Read the model definition and answer for the solid it produces. Units are mm, in the model's axes. Face numbers are marked on the shaded views. A direction names the side the tool comes from. Coordinates: 2 decimals unless noted, no trailing zeros. Loops run counter-clockwise (first coordinate to the right, second up) from the corner with the lowest first, then second, coordinate; pieces in that order, holes last. Notation, with made-up numbers: (-36.75, 72) - (-11.75, 72) arc R15 cw to (-11.75, 94) - close; hole circle Ø2 at (59.5, -12). An arc over 180 degrees is marked (long way). Use CSV: the item, a comma, the result in double quotes.
```python
from build123d import *

# Parameters (mm, degrees)
SKETCH3_W               = 6
SKETCH3_H               = 4
BOSS_EXTRUDE4_DEPTH     = 1
SKETCH7_W               = 2.025
SKETCH7_H               = 1
LPATTERN1_COUNT         = 5
LPATTERN1_PITCH         = 3
CUT_EXTRUDE2_DEPTH      = 15.053469323
CUT_EXTRUDE2_DEPTH_BACK = 15.053469323
CUT_EXTRUDE3_REACH      = 29.263
SKETCH6_R               = 1.5
SKETCH8_OUTSIDE_W       = 13.608
SKETCH8_OUTSIDE_H       = 12.19
SKETCH8_OUTSIDE_R       = 3
CUT_EXTRUDE4_DEPTH      = 15.017845865
CUT_EXTRUDE4_DEPTH_BACK = 15.017845865


with BuildPart() as part:
    # Sketch1 → Revolve5 (revolve)
    with BuildSketch(Plane.XY):
        Polygon((0, 13.5), (-2.5, 13.5), (-2.5, 13), (-2, 13), (-2, 5), (-2.25, 5), (-2.25, 4), (-2, 4), (-2, -13), (-2.5, -13), (-2.5, -13.5), (0, -13.5), align=None)
    revolve(axis=Axis((0, 13.5, 0), (0, -1, 0)))

    # Sketch3 → Boss-Extrude4 (add, symmetric)
    with BuildSketch(Plane.XY):
        with Locations((0, 4.5)):
            Rectangle(SKETCH3_W, SKETCH3_H)
    extrude(amount=BOSS_EXTRUDE4_DEPTH, both=True)

    # Sketch7 → Revolve7 (revolve)
    with BuildSketch(Plane.XY, mode=Mode.PRIVATE) as revolve7_sk:
        with Locations((-1.0125, -0.004180602)):
            Rectangle(SKETCH7_W, SKETCH7_H)
    revolve7 = revolve(revolve7_sk.sketch.rotate(Axis((0, 5, 0), (0, -1, 0)), 330), axis=Axis((0, 5, 0), (0, -1, 0)))

    # LPattern1: Revolve7 ×5
    with Locations(*[(0, -i * LPATTERN1_PITCH, 0) for i in range(1, LPATTERN1_COUNT)]):
        add(revolve7)

    # Sketch5 → Cut-Extrude2 (cut, two sides)
    with BuildSketch(Plane.XY) as cut_extrude2_sk:
        with BuildLine():
            Line((-1, 13.5), (-1, 10.5))
            ThreePointArc((-1, 10.5), (0, 9.5), (1, 10.5))
            Line((1, 10.5), (1, 13.5))
            Line((1, 13.5), (-1, 13.5))
        make_face()
        with BuildLine():
            Line((-1, -13.5), (-1, -10.5))
            ThreePointArc((-1, -10.5), (0, -9.5), (1, -10.5))
            Line((1, -10.5), (1, -13.5))
            Line((1, -13.5), (-1, -13.5))
        make_face()
    extrude(amount=CUT_EXTRUDE2_DEPTH, mode=Mode.SUBTRACT)
    extrude(cut_extrude2_sk.sketch, amount=-CUT_EXTRUDE2_DEPTH_BACK, mode=Mode.SUBTRACT)

    # Cut-Extrude3: up to this face of the body (flat: up to its plane)
    cut_extrude3_end = Plane(part.part.faces().sort_by_distance((-1.618726141, -13.5, 0))[0])
    # Sketch6 → Cut-Extrude3 (cut, up to the picked face)
    with BuildSketch(Plane(origin=(0, 13.5, 0), x_dir=(1, 0, 0), z_dir=(0, 1, 0)), mode=Mode.PRIVATE) as cut_extrude3_sk1:
        with Locations(Location((0, 0, 0), (0, 0, 228.189685104))):
            Circle(SKETCH6_R)
    cut_extrude3_tool1 = split(extrude(cut_extrude3_sk1.sketch, amount=-CUT_EXTRUDE3_REACH, mode=Mode.PRIVATE), bisect_by=cut_extrude3_end, keep=Keep.BOTH, mode=Mode.PRIVATE)
    add(cut_extrude3_tool1.solids().sort_by(Axis((0, 13.5, 0), (0, -1, 0)))[0], mode=Mode.SUBTRACT)

    # Sketch8 outside → Cut-Extrude4 (cut, two sides)
    with BuildSketch(Plane(origin=(0, 0, 0), x_dir=(1, 0, 0), z_dir=(0, 1, 0))) as cut_extrude4_sk:
        Rectangle(SKETCH8_OUTSIDE_W, SKETCH8_OUTSIDE_H)
        Circle(SKETCH8_OUTSIDE_R, mode=Mode.SUBTRACT)
    extrude(amount=CUT_EXTRUDE4_DEPTH, mode=Mode.SUBTRACT)
    extrude(cut_extrude4_sk.sketch, amount=-CUT_EXTRUDE4_DEPTH_BACK, mode=Mode.SUBTRACT)


solid = part.part
```
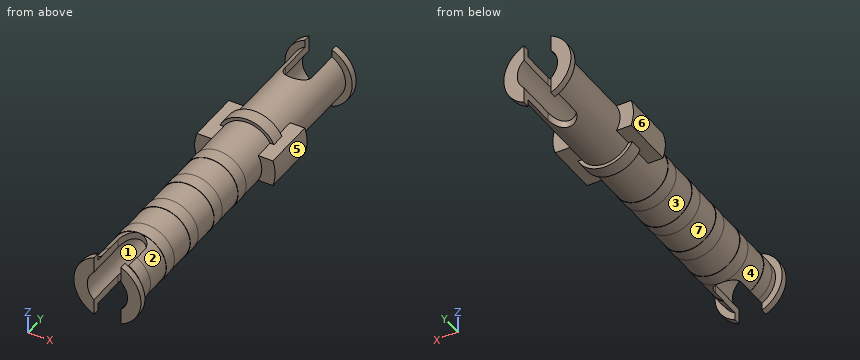
Q1. The part is cut by section A-A on y = 10.25. Determine the outline of the cut face in (x, z).
Reported:
outline,"(-0.97, -1.75) - (-0.97, -1.15) arc R1.5 cw to (-0.97, 1.15) - (-0.97, 1.75) arc R2 ccw to start; (0.97, -1.75) arc R2 ccw to (0.97, 1.75) - (0.97, 1.15) arc R1.5 cw to (0.97, -1.15) - close"
Q2. For a pull along Y with two mould halves and no side action, classify the marked faces 6 and 7 as +Y half, -Y half, draft (parallel to the pull), parting line (faces both ways), or undercut.
Reported:
face 6,"draft"
face 7,"undercut"
Q3. A tool of negligible diameter and unlimited length cuts with its end or side. For the marked faces 1, 2, 3, 4 and 5, from which of +Z, -Z, +X, -X, +Y, -Y can it reach the whole face along a straight path? Write none if from no direction.
Reported:
face 1,"+Y, -Y"
face 2,"+X"
face 3,"none"
face 4,"-X"
face 5,"+X, +Y, -Y"
Q4. Given P1, Ø0.9, axis at x = -2.5, y = 4.5, coming from the +Z side; P2, Ø1.3, axis at y = -11.5, z = -1.5, coming from the +X side; P3, Ø1.3, axis at y = -12, z = -1.5, coming from the -X side; P4, Ø2, axis at x = 0.5, z = -1, coming from the +Y side, each flat-ended and moving along its own axis, determine where each tip first touches the part or whether it passes through.
Reported:
P1,"stops at z = 1"
P2,"stops at x = 1.84"
P3,"stops at x = -1.84"
P4,"stops at y = 13.5"
Q5. Find the intervals of material crossed by probe 1 along Z at (x, y) = (0, -5); probe 2 along X at (y, z) = (4, 0), in increasing order. Write a range as [from, to].
Reported:
probe 1,"z = [-2, -1.5], [1.5, 2]"
probe 2,"x = [-3, -1.5], [1.5, 3]"
